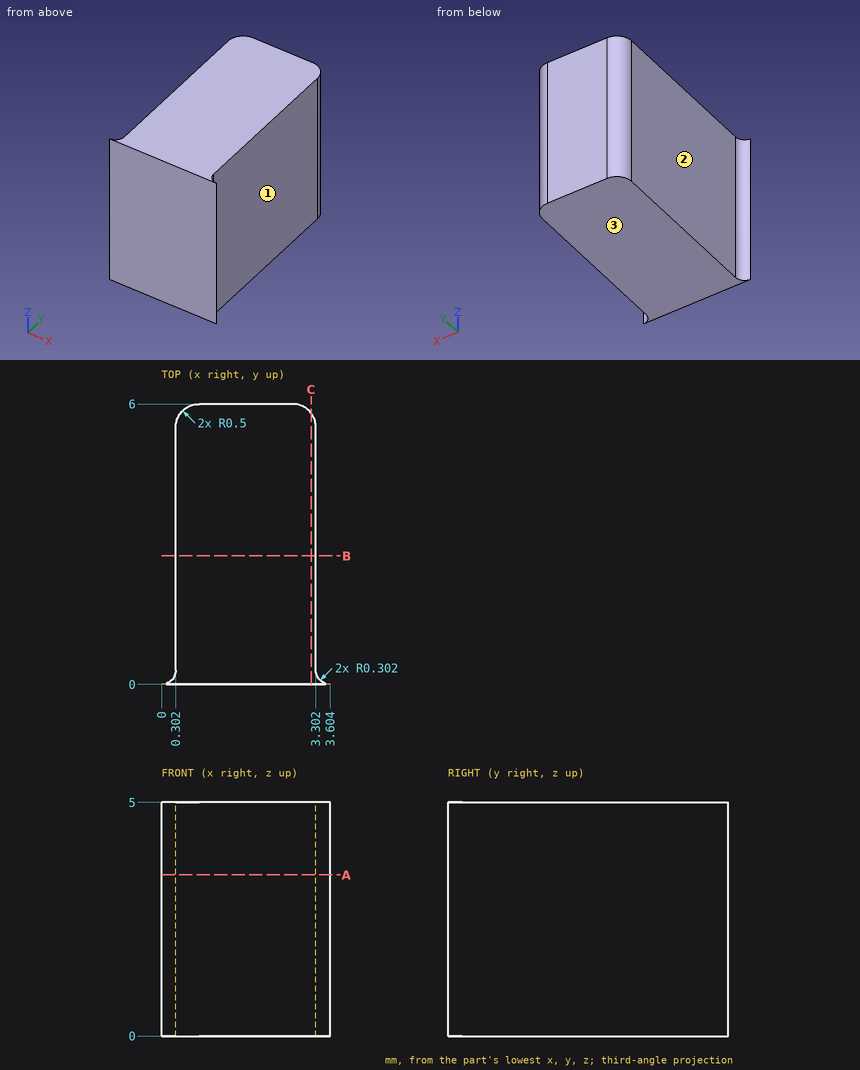
The drawing under review shows one solid part. Ordinate dimensions are in mm from its lowest x, y, z. A direction names the side the tool comes from. Give positions to 0.01 mm unless a question says otherwise; leave off trailing zeros. Loops run counter-clockwise (first coordinate to the right, second up) from the corner with the lowest first, then second, coordinate; pieces in that order, holes last. Notation, with made-up numbers: M 21.5,-7 L 72.5,-7 A11 cw 72.5,9 Z; hole C 5.25,-20.75 d7. An arc over 180 degrees is marked long. Return JSON: item names as keys, results as strings. Group by question number.
Item 1: For probe 1 along X at (y, z) = (2.25, 1.9); probe 2 along Y at (x, z) = (2.85, 0.3); probe 3 along Y at (x, z) = (0.4, 1.45), list the stretches that pass through material, from the lowest coordinate up.
Item 2: Insertion check: pin 1 Ø1.5 at (y, z) = (4, 3.5) entering from -X; pin 2 Ø2.5 at (y, z) = (3, 2.5) entering from +X. Each pin has a flat end and moves straight along its axis. Give the tip position at first contact, or say it passes through.
Item 3: We need section A-A (z = 3.45). Give the boundary of the cut face in (x, y), and give its area (3 significant figures).
Item 4: Tool access review of the marked faces 1, 2 and 3: name each direction out of +Z, -Z, +X, -X, +Y, -Y from which nothing blocks a thin tool from reaching the whole face with its end or side.
Item 5: We need section B-B (y = 2.75). Give the boundary of the cut face in (x, z), and give its area (3 significant figures).
Item 6: We need section C-C (x = 3.2). Give the boundary of the cut face in (y, z), and give its area (3 significant figures).
Output:
{
 "1": {"probe 1": "x = 0.3 to 3.3", "probe 2": "y = 0 to 6", "probe 3": "y = 0 to 5.8"},
 "2": {"pin 1": "stops at x = 0.3", "pin 2": "stops at x = 3.3"},
 "3": {"outline": "M 0,0 L 3.6,0 A0.3 cw 3.3,0.3 L 3.3,5.5 A0.5 ccw 2.8,6 L 0.8,6 A0.5 ccw 0.3,5.5 L 0.3,0.3 A0.3 cw Z", "area": "17.9 mm^2"},
 "4": {"face 1": "+Z, -Z, +X, +Y", "face 2": "+Z, -Z, -X, +Y", "face 3": "-Z, +X, -X, +Y, -Y"},
 "5": {"outline": "M 0.3,0 L 3.3,0 L 3.3,5 L 0.3,5 Z", "area": "15.0 mm^2"},
 "6": {"outline": "M 0,0 L 5.8,0 L 5.8,5 L 0,5 Z", "area": "29.0 mm^2"}
}
